```python
from build123d import *

# Parameters (mm, degrees)
SKETCH1_R           = 3.175
BOSS_EXTRUDE1_DEPTH = 28.575
CUT_EXTRUDE1_START  = -28.575
CUT_EXTRUDE1_DEPTH  = 3.175
BOSS_EXTRUDE2_START = 25.4
SKETCH3_R           = 3.175
BOSS_EXTRUDE2_DEPTH = 25.4


with BuildPart() as part:
    # Sketch1 → Boss-Extrude1 (new, symmetric)
    with BuildSketch(Plane(origin=(0, 0, 0), x_dir=(1, 0, 0), z_dir=(0, 1, 0))):
        with Locations(Location((0, 0, 0), (0, 0, 270))):
            Circle(SKETCH1_R)
    extrude(amount=BOSS_EXTRUDE1_DEPTH, both=True)

    # Sketch2 → Cut-Extrude1 (cut, symmetric)
    with BuildSketch(Plane(origin=(0, 28.575, 0), x_dir=(1, 0, 0), z_dir=(0, 1, 0)).offset(CUT_EXTRUDE1_START)):
        with BuildLine():
            Line((-1.905, 2.54), (-1.905, -2.54))
            ThreePointArc((-1.905, -2.54), (-3.175, 0), (-1.905, 2.54))
        make_face()
    extrude(amount=CUT_EXTRUDE1_DEPTH, both=True, mode=Mode.SUBTRACT)

    # Sketch3 → Boss-Extrude2 (add)
    with BuildSketch(Plane(origin=(0, 28.575, 0), x_dir=(1, 0, 0), z_dir=(0, 1, 0)).offset(BOSS_EXTRUDE2_START)):
        with Locations(Location((0, 0, 0), (0, 0, 270))):
            Circle(SKETCH3_R)
    extrude(amount=-BOSS_EXTRUDE2_DEPTH)


solid = part.part
```
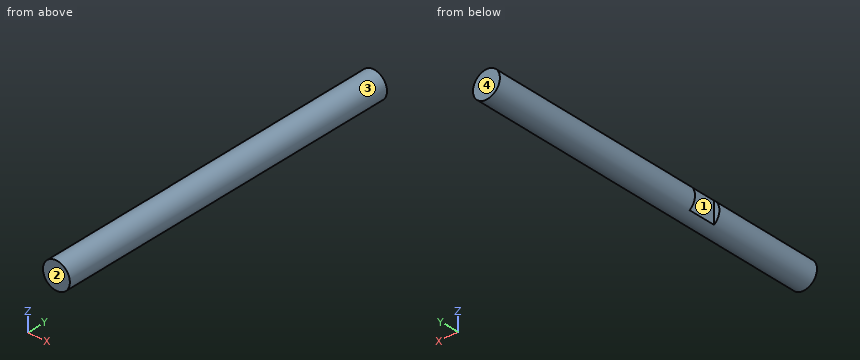
Here's how the part is built. I have some questions about the finished solid (model axes, mm). Face numbers are marked on the shaded views. Coordinates: 2 decimals unless noted, no trailing zeros. Order: outer loops, then holes, each group sorted by start corner. A loop starts at its lowest first (then second) coordinate and runs counter-clockwise, first axis right, second up. Notation, with made-up numbers: (46, 43) -> (61, 43) arc R21 cw to (61, 51) -> close; hole circle Ø8 at (-34, 5.25). An arc over 180 degrees is marked (long way). Return JSON: item names as keys, results as strings.
1) If I drill on probe 1 along Y at (x, z) = (-2.5, -0.25) (3 decimals); probe 2 along Z at (x, y) = (0.25, 44); probe 3 along X at (y, z) = (17, 1), over which ranges is the centre line in solid material (lowest first)?
Conclusion:
{"probe 1": "y = -28.575 to -3.175, 3.175 to 53.975", "probe 2": "z = -3.17 to 3.17", "probe 3": "x = -3.01 to 3.01"}
2) I'm going to push flat-ended pins straight in: P1, Ø3, axis at y = -18, z = -2.5, coming from the +X side; P2, Ø2, axis at y = 12, z = 2, coming from the -X side. Where does each tip first touch, or does it pass through?
Conclusion:
{"P1": "stops at x = 3.01", "P2": "stops at x = -3.01"}
3) If we section it at B-B on y = 5.5: List the corners of the cut face in (x, z) for me (3 decimals), plus the area to 3 significant figures.
Conclusion:
{"outline": "circle Ø6.35 at (0, 0)", "area": "31.7 mm²"}
4) If we section it at A-A on z = 0: List the corners of the cut face in (x, y) for me (3 decimals).
Conclusion:
{"outline": "(-3.175, -28.575) -> (3.175, -28.575) -> (3.175, 53.975) -> (-3.175, 53.975) -> (-3.175, 3.175) -> (-1.905, 3.175) -> (-1.905, -3.175) -> (-3.175, -3.175) -> close"}
5) Thinking about a two-plate mould opening in Y: for the marked faces 1, 2, 3 and 4, which applies, +Y half, -Y half, draft (parallel to the pull), parting line (faces both ways), or undercut?
Conclusion:
{"face 1": "undercut", "face 2": "-Y half", "face 3": "draft", "face 4": "+Y half"}
6) If we section it at C-C on x = 1.75: List the corners of the cut face in (y, z) for me (3 decimals), plus the area to 3 significant figures.
Conclusion:
{"outline": "(-28.575, -2.649) -> (53.975, -2.649) -> (53.975, 2.649) -> (-28.575, 2.649) -> close", "area": "437 mm²"}
